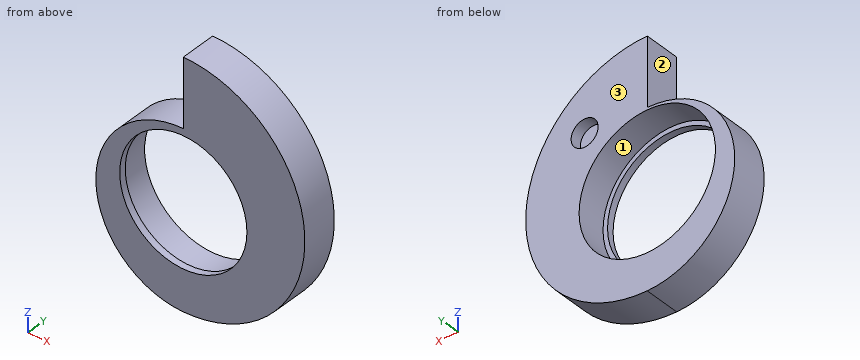
from build123d import *

# Parameters (mm, degrees)
F0_R     = 150
F1_DEPTH = 80
F2_R     = 150
F3_DEPTH = 65
F4_R     = 140
F5_DEPTH = 80.001
F6_R     = 29.726832
F7_DEPTH = 25


with BuildPart() as f1:
    # F0 (on Front) → F1 (new body)
    with BuildSketch(Plane.XZ):
        with BuildLine():
            Line((0, 305), (0, 155))
            ThreePointArc((0, 155), (-192.5, -37.5), (0, -230))
            ThreePointArc((0, -230), (267.5, 37.5), (0, 305))
        make_face()
        Circle(F0_R, mode=Mode.SUBTRACT)
        Circle(F0_R)
    extrude(amount=F1_DEPTH)

    # F2 (on Front) → F3 (cut)
    with BuildSketch(Plane.XZ):
        Circle(F2_R)
    extrude(amount=F3_DEPTH, mode=Mode.SUBTRACT)

    # F4 (on Front) → F5 (cut, through all)
    with BuildSketch(Plane.XZ):
        Circle(F4_R)
    extrude(amount=F5_DEPTH, mode=Mode.SUBTRACT)

    # F6 (on face) → F7 (cut)
    with BuildSketch(Plane(origin=(0, 0, 0), x_dir=(-1, 0, 0), z_dir=(0, 1, 0))):
        with Locations((-137.861013, 162.993148)):
            Circle(F6_R)
    extrude(amount=-F7_DEPTH, mode=Mode.SUBTRACT)


solid = f1.part
Read the model definition and answer for the solid it produces. Units are mm, in the model's axes. Face numbers are marked on the shaded views. Give positions to 0.01 mm unless a question says otherwise; leave off trailing zeros. Write each loop counter-clockwise with the first axis right and the second up, starting at its lowest first coordinate (ties: lowest second). Pieces come first, ordered by that corner, then holes. Notation, with made-up numbers: (52.25, 70.5) -> (64.25, 70.5) arc R18 ccw to (64.25, 75.5) -> close; hole circle Ø2 at (-30, -15). An arc over 180 degrees is marked (long way). Answer as a JSON object with one key per item and string values. Group by question number.
1) Each of these flat-tipped pins is pushed along its axis until it touches: P1, Ø8, axis at x = 48, y = -65, coming from the -Z side; P2, Ø1.5, axis at x = -37.5, y = -11.5, coming from the +Z side; P3, Ø1, axis at x = 174, y = -60, coming from the -Z side. Where does it stop, or does it pass through?
2) The mould has two halves that part along X. Classify the marked faces 1, 2 and 3: +X half, -X half, draft (parallel to the pull), parting line (faces both ways), or undercut.
3) Find section A-A (z = 37.5). Write down the section's boundary in (x, y), and give its area (3 significant figures).
4) Find section D-D (x = 190.5). Write down the section's boundary in (y, z).
5) Find section C-C (x = -67.5). Write down the section's boundary in (y, z).
6) Consider L1, parallel to Y at x = 43.5, z = 134; L2, parallel to Z at x = -116, y = -35.5; L3, parallel to Z at x = 34.5, y = -48.5. Determine where each line is inside the solid, lowest interval first. Write a range as from..to.
7) Find section B-B (x = 128). Write down the section's boundary in (y, z), and give its area (3 significant figures).
Values follow:
{
 "1": {"P1": "stops at z = -226.36", "P2": "stops at z = 151.46", "P3": "stops at z = -166.1"},
 "2": {"face 1": "undercut", "face 2": "-X half", "face 3": "draft"},
 "3": {"outline": "(-177.29, -80) -> (-134.88, -80) -> (-134.88, -65) -> (-145.24, -65) -> (-145.24, 0) -> (-177.29, 0) -> close; (134.88, -80) -> (267.5, -80) -> (267.5, 0) -> (145.24, 0) -> (145.24, -65) -> (134.88, -65) -> close", "area": "12,700 mm2"},
 "4": {"outline": "(-80, -150.29) -> (0, -150.29) -> (0, 225.29) -> (-80, 225.29) -> close"},
 "5": {"outline": "(-80, -217.78) -> (0, -217.78) -> (0, -133.95) -> (-65, -133.95) -> (-65, -122.65) -> (-80, -122.65) -> close; (-80, 122.65) -> (-65, 122.65) -> (-65, 133.95) -> (0, 133.95) -> (0, 142.78) -> (-80, 142.78) -> close"},
 "6": {"L1": "y = -80..-65", "L2": "z = -191.12..-95.1, 95.1..116.12", "L3": "z = -227.77..-145.98, 145.98..302.77"},
 "7": {"outline": "(-80, -197.39) -> (0, -197.39) -> (0, -78.2) -> (-65, -78.2) -> (-65, -56.71) -> (-80, -56.71) -> close; (-80, 56.71) -> (-65, 56.71) -> (-65, 78.2) -> (0, 78.2) -> (0, 134.95) -> (-25, 134.95) -> (-25, 191.04) -> (0, 191.04) -> (0, 272.39) -> (-80, 272.39) -> close", "area": "24,300 mm2"}
}
